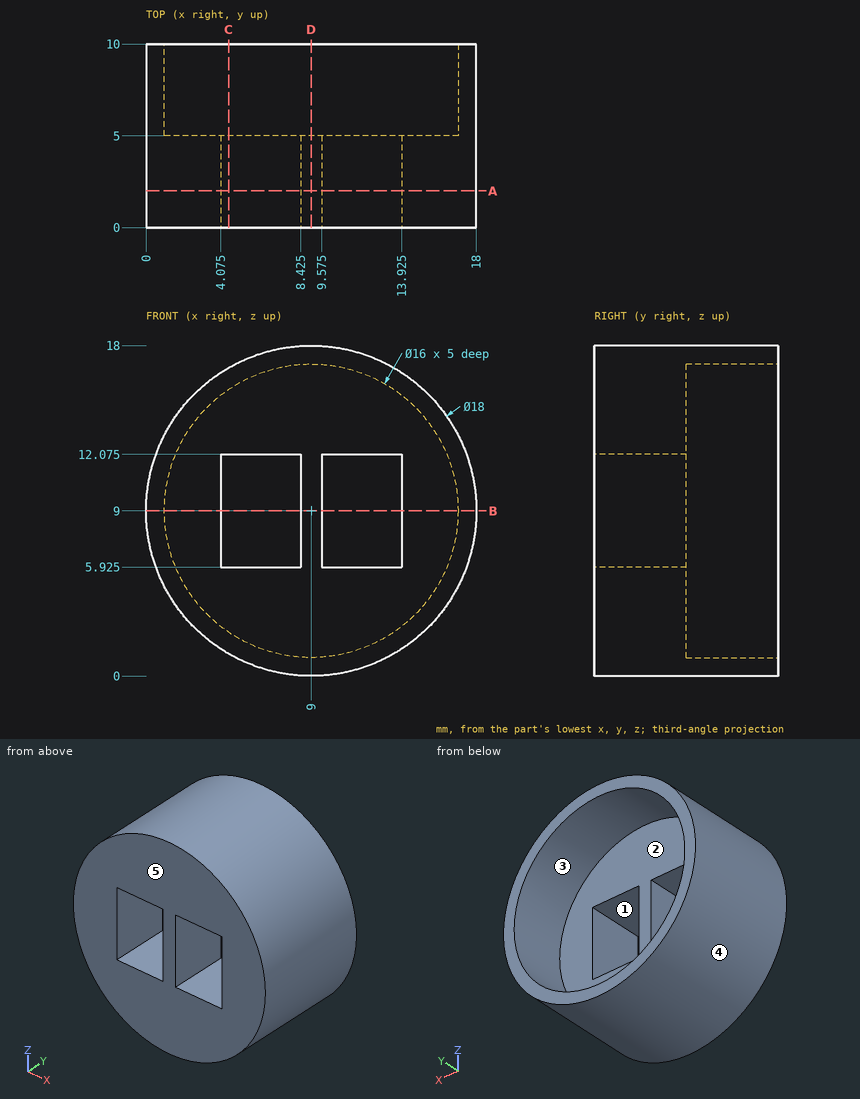
Input: dimensioned drawing with shaded views. Units: mm. Origin: part minimum x, y, z. A direction names the side the tool comes from. Round coordinates to 2 decimals unless told otherwise and drop trailing zeros. Loops run counter-clockwise (first coordinate to the right, second up) from the corner with the lowest first, then second, coordinate; pieces in that order, holes last. Notation, with made-up numbers: (87, 53) -> (125, 53) arc R19 cw to (125, 59) -> close; hole circle Ø10 at (60.25, -19.5). An arc over 180 degrees is marked (long way). Answer as a JSON object with one key per item and string values. Group by question number.
Q1. Section query A-A (y = 2). Output: boundary loops of the cut face in (x, z) (3 decimals).
Q2. Contact query for flat-ended pins moving along their axis: P1, Ø5, axis at x = 5.5, y = 1.5, coming from the +Z side; P2, Ø2.5, axis at y = 1.5, z = 10.5, coming from the +X side; P3, Ø1.5, axis at y = 3.5, z = 8, coming from the -X side; P4, Ø1, axis at x = 3, z = 12, coming from the -Y side. Output: stop coordinate, or through.
Q3. Section query B-B (z = 9). Output: boundary loops of the cut face in (x, y) (3 decimals), plus the area to 3 significant figures.
Q4. Section query D-D (x = 9). Output: boundary loops of the cut face in (y, z), plus the area to 3 significant figures.
Q5. Section query C-C (x = 4.5). Output: boundary loops of the cut face in (y, z) (3 decimals).
Q6. Mould query, pull axis X, two halves, no side actions, for the marked faces 3, 4 and 5. Classes: pulls with the +X half, pulls with the -X half, needs draft (parallel to the pull), parting line crosses it, or undercut.
Q7. Access query for the marked faces 1 and 2. Directions: +Z, -Z, +X, -X, +Y, -Y. A direction counts if a zero-diameter tool reaches every point of the face in a straight line with its end or side. Return the directions, or none.
Q8. Ray query, line 1 (Z direction, x = 9, y = 6.35); line 2 (Z direction, x = 14.5, y = 7.5). Return the intervals inside material, ascending. Write a range as from..to.
Completed:
{
 "1": {"outline": "circle Ø18 at (9, 9); hole (4.075, 5.925) -> (8.425, 5.925) -> (8.425, 12.075) -> (4.075, 12.075) -> close; hole (9.575, 5.925) -> (13.925, 5.925) -> (13.925, 12.075) -> (9.575, 12.075) -> close"},
 "2": {"P1": "z = 17.94", "P2": "x = 18", "P3": "x = 0", "P4": "y = 0"},
 "3": {"outline": "(0, 0) -> (4.075, 0) -> (4.075, 5) -> (1, 5) -> (1, 10) -> (0, 10) -> close; (8.425, 0) -> (9.575, 0) -> (9.575, 5) -> (8.425, 5) -> close; (13.925, 0) -> (18, 0) -> (18, 10) -> (17, 10) -> (17, 5) -> (13.925, 5) -> close", "area": "56.5 mm²"},
 "4": {"outline": "(0, 0) -> (10, 0) -> (10, 1) -> (5, 1) -> (5, 17) -> (10, 17) -> (10, 18) -> (0, 18) -> close", "area": "100 mm²"},
 "5": {"outline": "(0, 1.206) -> (10, 1.206) -> (10, 2.386) -> (5, 2.386) -> (5, 5.925) -> (0, 5.925) -> close; (0, 12.075) -> (5, 12.075) -> (5, 15.614) -> (10, 15.614) -> (10, 16.794) -> (0, 16.794) -> close"},
 "6": {"face 3": "undercut", "face 4": "parting line crosses it", "face 5": "needs draft"},
 "7": {"face 1": "+Y, -Y", "face 2": "+Y"},
 "8": {"line 1": "0..1, 17..18", "line 2": "1.88..3.19, 14.81..16.12"}
}
